Verification items for the finished model (mm, model axes). Give positions to 0.01 mm unless a question says otherwise; leave off trailing zeros. Loops run counter-clockwise (first coordinate to the right, second up) from the corner with the lowest first, then second, coordinate; pieces in that order, holes last. Notation, with made-up numbers: (16.25, 89.5) - (53.25, 89.5) arc R15 cw to (53.25, 100.5) - close; hole circle Ø3 at (75.25, -3.75). An arc over 180 degrees is marked (long way). Answer in a Markdown table with one row per item.
```python
from build123d import *

# Parameters (mm, degrees)
SKETCH1_W           = 14.51987794
SKETCH1_H           = 27.697484205
BOSS_EXTRUDE1_DEPTH = 3


with BuildPart() as part:
    # Sketch1 → Boss-Extrude1 (new body)
    with BuildSketch(Plane.XY):
        Polygon((10.672922398, 975.073069212), (10.566207631, 1059.617843106), (489.608405369, 1059.006658046), (489.715120136, 974.461884152), align=None)
        with Locations((90.428871138, 1017.342955032)):
            Rectangle(SKETCH1_W, SKETCH1_H, mode=Mode.SUBTRACT)
        Polygon((402.675989281, 1031.301508945), (417.19585566, 1031.283185961), (417.160903536, 1003.585723809), (402.641037157, 1003.604046793), align=None, mode=Mode.SUBTRACT)
    extrude(amount=BOSS_EXTRUDE1_DEPTH)


solid = part.part
```
Q1. Go/stop test with flat-tipped pins: P1, Ø1.5, axis at x = 92.5, z = 2, coming from the +Y side; P2, Ø0.9, axis at y = 1020.5, z = 1.5, coming from the -X side (3 decimals). Record where each tip stops, or that it passes through.
Completed:
| item | result |
|---|---|
| P1 | y = 1059.51 |
| P2 | x = 10.615 |
Q2. Thickness scan on line 1 (X direction, y = 1008.5, z = 2.35); line 2 (X direction, y = 980.5, z = 2.55). Record the ranges inside material, lowest first.
Completed:
| item | result |
|---|---|
| line 1 | 10.63 to 83.17, 97.69 to 402.65, 417.17 to 489.67 |
| line 2 | 10.67 to 489.71 |
Q3. Sectioned sample at A-A (z = 0.95). Record the cut outline in (x, y), and give its area (3 significant figures).
Completed:
| item | result |
|---|---|
| outline | (10.57, 1059.62) - (10.67, 975.07) - (489.72, 974.46) - (489.61, 1059.01) - close; hole (83.17, 1003.49) - (97.69, 1003.49) - (97.69, 1031.19) - (83.17, 1031.19) - close; hole (402.64, 1003.6) - (417.16, 1003.59) - (417.2, 1031.28) - (402.68, 1031.3) - close |
| area | 39,700 mm^2 |
Q4. Sectioned sample at B-B (y = 1014). Record the cut outline in (x, z).
Completed:
| item | result |
|---|---|
| outline | (10.62, 0) - (83.17, 0) - (83.17, 3) - (10.62, 3) - close; (97.69, 0) - (402.65, 0) - (402.65, 3) - (97.69, 3) - close; (417.17, 0) - (489.67, 0) - (489.67, 3) - (417.17, 3) - close |
